Work out the finished part from the listing and answer in its coordinate system (mm). Coordinates: 2 decimals unless noted, no trailing zeros. Loops run counter-clockwise (first coordinate to the right, second up) from the corner with the lowest first, then second, coordinate; pieces in that order, holes last. Notation, with made-up numbers: (27, -36.5) -> (45, -36.5) arc R6 ccw to (45, -26.5) -> close; hole circle Ø10 at (46.25, 79). An arc over 180 degrees is marked (long way). One line per question, with ' | ' between items.
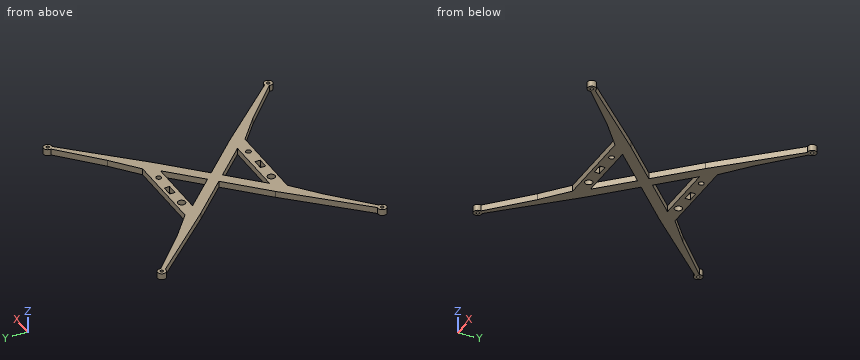
```python
from build123d import *

# Parameters (mm, degrees)
F0_R         = 4
F1_DEPTH     = 6
F3_DEPTH     = 6
F4_R         = 1.5
F5_DEPTH     = 6.001
F6_COUNT     = 4
F8_W         = 85
F8_H         = 12
F9_DEPTH     = 6
F10_R        = 3.55
F10_R_2      = 2.5
F10_W        = 10
F10_H        = 5
F11_DEPTH    = 6.001
F12_C1_SIZE2 = 3
F12_C1_SIZE  = 30
F12_C2_SIZE2 = 30
F12_C2_SIZE  = 3
F12_C3_SIZE2 = 3
F12_C3_SIZE  = 30
F12_C4_SIZE2 = 30
F12_C4_SIZE  = 3


# Not quite as in the source:
# - a pattern or mirror of a feature is missing from the dataset's text; its kind, count and spacing are read off the source's solid


with BuildPart() as f1:
    # F0 (on Top) → F1 (new body)
    with BuildSketch(Plane.XY):
        with Locations((-104.5, 104.5)):
            Circle(F0_R)
    extrude(amount=F1_DEPTH)

    # F2 (on Top) → F3 (join, through all)
    with BuildSketch(Plane.XY):
        Polygon((-7.0710678119, 0), (0, 0), (0, 7.0710678119), (-35.3553390593, 42.4264068712), (-100.6362966948, 103.4647238196), (-103.4647238196, 100.6362966948), (-42.4264068712, 35.3553390593), align=None)
    extrude(amount=F3_DEPTH)

    # F4 (on face) → F5 (cut, through all)
    with BuildSketch(Plane.XY.offset(6)):
        with Locations((-104.5, 104.5)):
            Circle(F4_R)
    extrude(amount=-F5_DEPTH, mode=Mode.SUBTRACT)


with BuildPart() as f6_1:
    # F6: instance of F1
    add(f1.part.rotate(Axis((0, 0, 3), (0, 0, -1)), 1 * 360 / F6_COUNT))


with BuildPart() as f6_2:
    # F6: instance of F1
    add(f1.part.rotate(Axis((0, 0, 3), (0, 0, -1)), 2 * 360 / F6_COUNT))


with BuildPart() as f6_3:
    # F6: instance of F1
    add(f1.part.rotate(Axis((0, 0, 3), (0, 0, -1)), 3 * 360 / F6_COUNT))


with BuildPart() as f1_1:
    add(f1.part)

    # F7: union F6_1, F6_2, F6_3
    add(f6_1.part)
    add(f6_2.part)
    add(f6_3.part)

    # F8 (on Top) → F9 (join, through all)
    with BuildSketch(Plane.XY):
        with Locations((0, 42.5)):
            Rectangle(F8_W, F8_H)
    f9 = extrude(amount=F9_DEPTH)

    # F9_copies: F9 across plane
    add(f9.mirror(Plane(origin=(0, 0, 0), x_dir=(0, 0, -1), z_dir=(0, -1, 0))))

    # F10 (on face) → F11 (cut, through all)
    with BuildSketch(Plane.XY.offset(6)):
        with Locations((-21, 42.5)):
            Circle(F10_R)
        with Locations((21, 42.5)):
            Circle(F10_R_2)
        with Locations((0, 43)):
            Rectangle(F10_W, F10_H)
    f11 = extrude(amount=-F11_DEPTH, mode=Mode.SUBTRACT)

    # F11_copies: F11 across plane
    add(f11.mirror(Plane(origin=(0, 0, 0), x_dir=(0, 0, -1), z_dir=(0, -1, 0))), mode=Mode.SUBTRACT)

    # F12: chamfer of 3 x 30 on 4 edges, made by hand

    # F12_c1
    f12_c1_edges = [f1_1.edges().sort_by_distance(p)[0] for p in [
        (-41.8510944399, 48.5, 3),
    ]]
    f12_c1_side = f1_1.faces().sort_by_distance((-41.8949210948, 48.5409783396, 3))[0]
    chamfer(f12_c1_edges, length=F12_C1_SIZE, length2=F12_C1_SIZE2, reference=f12_c1_side)

    # F12_c2
    f12_c2_edges = [f1_1.edges().sort_by_distance(p)[0] for p in [
        (41.8510944399, 48.5, 3),
    ]]
    f12_c2_side = f1_1.faces().sort_by_distance((41.7910944399, 48.5, 3))[0]
    chamfer(f12_c2_edges, length=F12_C2_SIZE, length2=F12_C2_SIZE2, reference=f12_c2_side)

    # F12_c3
    f12_c3_edges = [f1_1.edges().sort_by_distance(p)[0] for p in [
        (41.8510944399, -48.5, 3),
    ]]
    f12_c3_side = f1_1.faces().sort_by_distance((41.8949210948, -48.5409783396, 3))[0]
    chamfer(f12_c3_edges, length=F12_C3_SIZE, length2=F12_C3_SIZE2, reference=f12_c3_side)

    # F12_c4
    f12_c4_edges = [f1_1.edges().sort_by_distance(p)[0] for p in [
        (-41.8510944399, -48.5, 3),
    ]]
    f12_c4_side = f1_1.faces().sort_by_distance((-41.7910944399, -48.5, 3))[0]
    chamfer(f12_c4_edges, length=F12_C4_SIZE, length2=F12_C4_SIZE2, reference=f12_c4_side)


solid = f1_1.part
```
1) Flat-ended cylindrical pins translate along their axes: pin 1 (1.5 mm diameter, centred on y = -43.5, z = 4, fed in from +X); pin 2 (4 mm diameter, centred on x = -74, y = 81.5, fed in from +Z); pin 3 (1.8 mm diameter, centred on x = -12.5, z = 3, fed in from +Y); pin 4 (1.8 mm diameter, centred on x = -12, z = 2.5, fed in from -Y). Find the tip coordinate at first contact, or state that the pin passes through.
Check values:
pin 1: stops at x = 50.74 | pin 2: passes through | pin 3: stops at y = 48.5 | pin 4: stops at y = -48.5
2) Find the intervals of material crossed by line 1 along X through (y, z) = (104.5, 1.85); line 2 along Y through (x, z) = (-16.5, 4.9); line 3 along Y through (x, z) = (-16, 2.75), in increasing order.
Check values:
line 1: x = -108.5 to -106, -103 to -100.5, 100.5 to 103, 106 to 108.5 | line 2: y = -48.5 to -36.5, -23.57 to -9.43, 9.43 to 23.57, 36.5 to 48.5 | line 3: y = -48.5 to -36.5, -23.07 to -8.93, 8.93 to 23.07, 36.5 to 48.5
3) Find section A-A (y = 76.5). Write down the section's boundary in (x, z), plus the area to 3 significant figures.
Check values:
outline: (-80.9, 0) -> (-71.8, 0) -> (-71.8, 6) -> (-80.9, 6) -> close; (71.8, 0) -> (80.9, 0) -> (80.9, 6) -> (71.8, 6) -> close | area: 109 mm^2
4) Find section D-D (z = 3.6). State how many separate pieces and enclosed holes the cut face has, plus the area to 3 significant figures.
Check values:
separate pieces: 1 | enclosed holes: 12 | area: 6,380 mm^2
5) Find section B-B (x = 21). Write down the section's boundary in (y, z), plus the area to 3 significant figures.
Check values:
outline: (-48.5, 0) -> (-45, 0) -> (-45, 6) -> (-48.5, 6) -> close; (-40, 0) -> (-36.5, 0) -> (-36.5, 6) -> (-40, 6) -> close; (-28.07, 0) -> (-13.93, 0) -> (-13.93, 6) -> (-28.07, 6) -> close; (13.93, 0) -> (28.07, 0) -> (28.07, 6) -> (13.93, 6) -> close; (36.5, 0) -> (40, 0) -> (40, 6) -> (36.5, 6) -> close; (45, 0) -> (48.5, 0) -> (48.5, 6) -> (45, 6) -> close | area: 254 mm^2
6) Find section C-C (x = -59). Write down the section's boundary in (y, z), plus the area to 3 significant figures.
Check values:
outline: (-65.07, 0) -> (-53.08, 0) -> (-53.08, 6) -> (-65.07, 6) -> close; (53.08, 0) -> (65.07, 0) -> (65.07, 6) -> (53.08, 6) -> close | area: 144 mm^2
